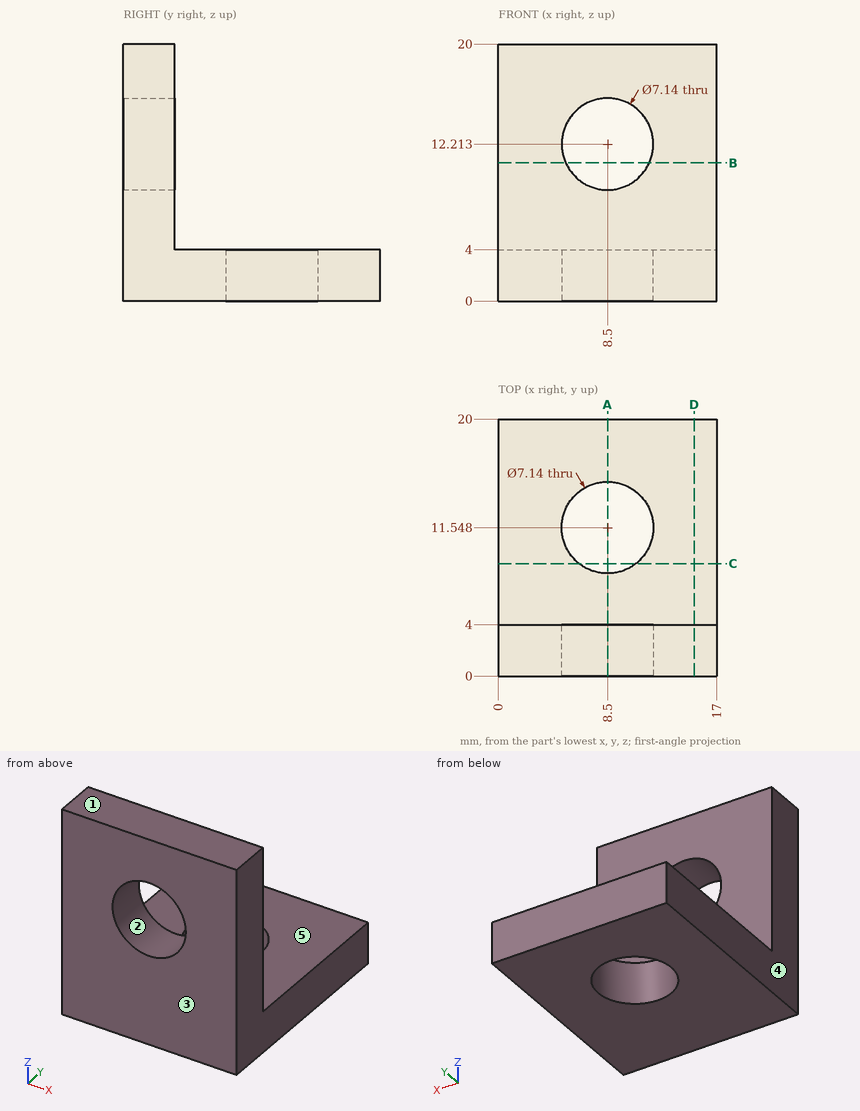
Input: dimensioned drawing with shaded views. Units: mm. Origin: part minimum x, y, z. A direction names the side the tool comes from. Coordinates: 2 decimals unless noted, no trailing zeros. Loops run counter-clockwise (first coordinate to the right, second up) from the corner with the lowest first, then second, coordinate; pieces in that order, holes last. Notation, with made-up numbers: (76, 36.25) -> (114, 36.25) arc R23 ccw to (114, 63.25) -> close; hole circle Ø9 at (1, 34.5). An arc over 180 degrees is marked (long way). Use a Markdown table: item, result. Add a question column.
(1) Section query A-A, the plane x = 8.5. Return loops of the section in (y, z).
(2) Section query D-D, the plane x = 15.25. Return loops of the section in (y, z).
(3) Access query for the marked faces 4 and 5. Directions: +Z, -Z, +X, -X, +Y, -Y. A direction counts if a zero-diameter tool reaches every point of the face in a straight line with its end or side. Return the directions, or none.
(4) Section query C-C, the plane y = 8.75. Return loops of the section in (x, z).
(5) Line query: line 1 along Z through (x, y) = (8.5, 2.3); line 2 along Y through (x, z) = (8.5, 1.3); line 3 along Y through (x, z) = (13.5, 16). Output: solid intervals per line, ascending.
(6) Section query B-B, the plane z = 10.75. Return loops of the section in (x, y).
(7) Mould query, pull axis Z, two halves, no side actions, for the marked faces 1, 2 and 3. Classes: pulls with the +Z half, pulls with the -Z half, needs draft (parallel to the pull), parting line crosses it, or undercut.
(8) Pin query (flat end, axial travel): pin 1 Ø10 at (x, z) = (2.5, 14.5) entering from +Y; pin 2 Ø1 at (x, y) = (10.5, 9) entering from +Z. Return the tip coordinate at first contact, or that it passes through.
Answer:
| question | item | result |
|---|---|---|
| 1 | outline | (0, 0) -> (7.98, 0) -> (7.98, 4) -> (4, 4) -> (4, 8.64) -> (0, 8.64) -> close; (0, 15.78) -> (4, 15.78) -> (4, 20) -> (0, 20) -> close; (15.12, 0) -> (20, 0) -> (20, 4) -> (15.12, 4) -> close |
| 2 | outline | (0, 0) -> (20, 0) -> (20, 4) -> (4, 4) -> (4, 20) -> (0, 20) -> close |
| 3 | face 4 | +Z, -Z, -X, +Y, -Y |
| 3 | face 5 | +Z, +X, -X, +Y |
| 4 | outline | (0, 0) -> (6.28, 0) -> (6.28, 4) -> (0, 4) -> close; (10.72, 0) -> (17, 0) -> (17, 4) -> (10.72, 4) -> close |
| 5 | line 1 | z = 0 to 8.64, 15.78 to 20 |
| 5 | line 2 | y = 0 to 7.98, 15.12 to 20 |
| 5 | line 3 | y = 0 to 4 |
| 6 | outline | (0, 0) -> (5.24, 0) -> (5.24, 4) -> (0, 4) -> close; (11.76, 0) -> (17, 0) -> (17, 4) -> (11.76, 4) -> close |
| 7 | face 1 | pulls with the +Z half |
| 7 | face 2 | undercut |
| 7 | face 3 | needs draft |
| 8 | pin 1 | stops at y = 4 |
| 8 | pin 2 | stops at z = 4 |
